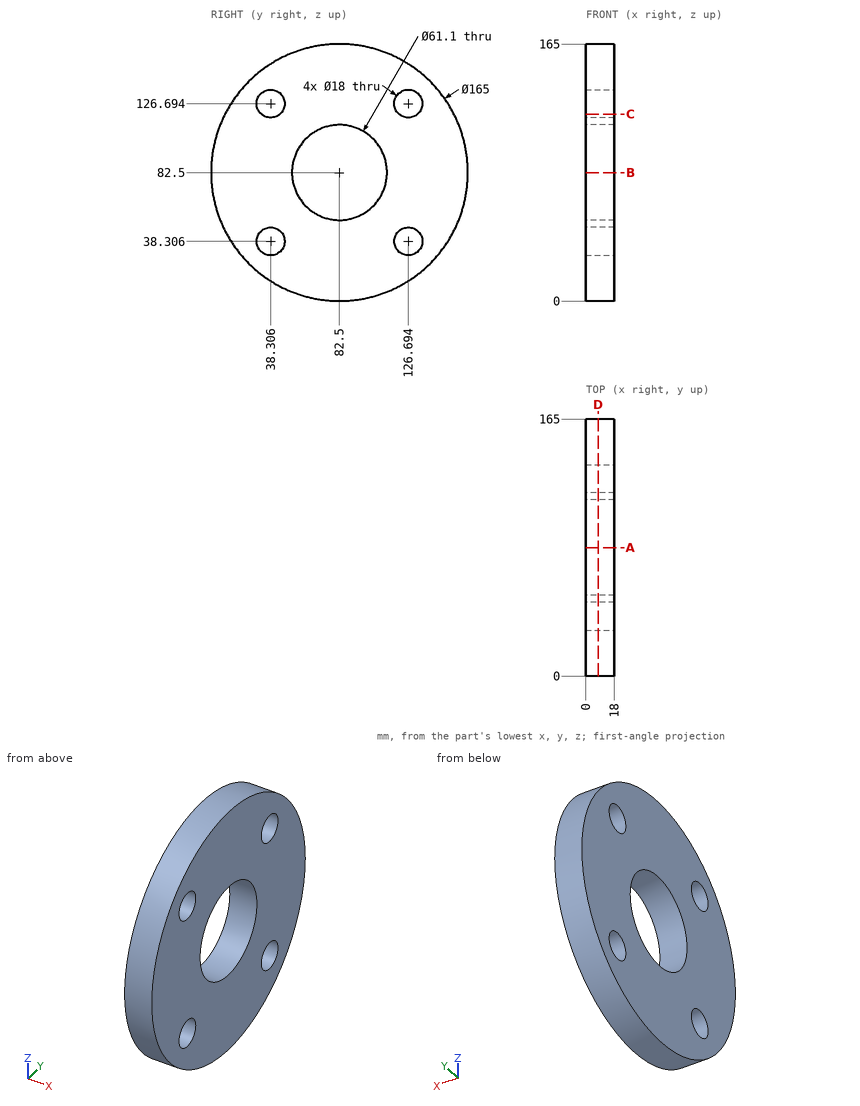
Source: three-view drawing plus pictorial views. Frame: mm from the lowest corner of the part. Give positions to 0.01 mm unless a question says otherwise; leave off trailing zeros. Loops run counter-clockwise (first coordinate to the right, second up) from the corner with the lowest first, then second, coordinate; pieces in that order, holes last. Notation, with made-up numbers: (-3.5, 16.25) -> (44.5, 16.25) arc R23 ccw to (44.5, 39.25) -> close; hole circle Ø3 at (8, 68.25). An arc over 180 degrees is marked (long way). Put each result on its own line as item: value. Start each with the question number.
1) Material intervals for probe 1 along Z at (x, y) = (13.75, 122) (1 decimal); probe 2 along Y at (x, z) = (3.25, 124.5) (1 decimal); probe 3 along Z at (x, y) = (15, 98), sorted ascending.
2) Cut plane C-C (z = 120). Return loops of the section in (x, y) (1 decimal), then the cut area to 3 significant figures.
3) Cut plane A-A (y = 82.5). Return loops of the section in (x, z), then the cut area to 3 significant figures.
4) Cut plane D-D (x = 7.75). Return loops of the section in (y, z), then the cut area to 3 significant figures.
5) Contact query for flat-ended pins moving along their axis: P1, Ø1, axis at x = 3, z = 65, coming from the -Y side; P2, Ø8, axis at x = 2.5, y = 62.5, coming from the +Z side; P3, Ø1.5, axis at x = 5.5, z = 17, coming from the -Y side (1 decimal). Output: stop coordinate, or through.
Results are:
1. probe 1: z = 10.1 to 30.6, 46 to 119, 134.4 to 154.9
1. probe 2: y = 11.5 to 29.6, 47 to 118, 135.4 to 153.5
1. probe 3: z = 1.47 to 56.17, 108.83 to 163.53
2. outline: (0, 9) -> (18, 9) -> (18, 32.3) -> (0, 32.3) -> close; (0, 44.3) -> (18, 44.3) -> (18, 120.7) -> (0, 120.7) -> close; (0, 132.7) -> (18, 132.7) -> (18, 156) -> (0, 156) -> close
2. area: 2,210 mm2
3. outline: (0, 0) -> (18, 0) -> (18, 51.95) -> (0, 51.95) -> close; (0, 113.05) -> (18, 113.05) -> (18, 165) -> (0, 165) -> close
3. area: 1,870 mm2
4. outline: circle Ø165 at (82.5, 82.5); hole circle Ø18 at (38.31, 38.31); hole circle Ø18 at (38.31, 126.69); hole circle Ø61.1 at (82.5, 82.5); hole circle Ø18 at (126.69, 38.31); hole circle Ø18 at (126.69, 126.69)
4. area: 17,400 mm2
5. P1: stops at y = 1.77
5. P2: stops at z = 163.43
5. P3: stops at y = 31.4
